Could you check a few things on this model? Use its own coordinates, in mm. Face numbers are marked on the shaded views. Round coordinates to 2 decimals unless told otherwise and drop trailing zeros. Loops run counter-clockwise (first coordinate to the right, second up) from the corner with the lowest first, then second, coordinate; pieces in that order, holes last. Notation, with made-up numbers: (50, 12.25) -> (102, 12.25) arc R19 cw to (102, 40.25) -> close; hole circle Ø4 at (20.25, -36.5). An arc over 180 degrees is marked (long way). One line per item, written item: value.
```python
from build123d import *

# Parameters (mm, degrees)
F0_W     = 67.8
F0_H     = 42
F0_R     = 0.75
F0_W_2   = 2
F0_H_2   = 0.6
F1_DEPTH = 5.3
F2_DEPTH = 1.5
F3_DEPTH = 3.1
F5_DEPTH = 3.3
F7_DEPTH = 1.3
F9_DEPTH = 1.8
F10_SIZE = 0.2


with BuildPart() as f1:
    # F0 (on Top) → F1 (new body)
    with BuildSketch(Plane.XY):
        Rectangle(F0_W, F0_H)
        with Locations((-32.9, -20)):
            Circle(F0_R, mode=Mode.SUBTRACT)
        with Locations((-23.9, -19.7)):
            Rectangle(F0_W_2, F0_H_2, mode=Mode.SUBTRACT)
        with Locations((23.9, -19.7)):
            Rectangle(F0_W_2, F0_H_2, mode=Mode.SUBTRACT)
        with Locations((32.9, -20)):
            Circle(F0_R, mode=Mode.SUBTRACT)
        with Locations((-32.9, 20)):
            Circle(F0_R, mode=Mode.SUBTRACT)
        with Locations((32.9, 20)):
            Circle(F0_R, mode=Mode.SUBTRACT)
        with Locations((32.9, 20)):
            Circle(F0_R)
        with Locations((32.9, -20)):
            Circle(F0_R)
        with Locations((-32.9, 20)):
            Circle(F0_R)
        with Locations((-32.9, -20)):
            Circle(F0_R)
        with Locations((-23.9, -19.7)):
            Rectangle(F0_W_2, F0_H_2)
        with Locations((23.9, -19.7)):
            Rectangle(F0_W_2, F0_H_2)
    extrude(amount=F1_DEPTH)

    # F0 (on Top) → F2 (join)
    with BuildSketch(Plane.XY):
        with Locations((-32.9, -20)):
            Circle(F0_R)
        with Locations((32.9, -20)):
            Circle(F0_R)
        with Locations((32.9, 20)):
            Circle(F0_R)
        with Locations((-32.9, 20)):
            Circle(F0_R)
    extrude(amount=-F2_DEPTH)

    # F0 (on Top) → F3 (join)
    with BuildSketch(Plane.XY):
        with Locations((-23.9, -19.7)):
            Rectangle(F0_W_2, F0_H_2)
        with Locations((23.9, -19.7)):
            Rectangle(F0_W_2, F0_H_2)
    extrude(amount=-F3_DEPTH)

    # F4 (on face) → F5 (cut)
    with BuildSketch(Plane.XY.offset(5.3)):
        Polygon((33, 17), (33, 20), (29.9, 20), (29.9, 21), (-29.9, 21), (-29.9, 20), (-33, 20), (-33, 17), (-33.9, 17), (-33.9, -17), (-33, -17), (-33, -20), (-29.9, -20), (-29.9, -21), (29.9, -21), (29.9, -20), (33, -20), (33, -17), (33.9, -17), (33.9, 17), align=None)
    extrude(amount=-F5_DEPTH, mode=Mode.SUBTRACT)

    # F6 (on face) → F7 (join)
    with BuildSketch(Plane.XY.offset(2)):
        Polygon((33, 17), (33, 20), (29.9, 20), (-29.9, 20), (-33, 20), (-33, 17), (-33, -17), (-33, -20), (-29.9, -20), (29.9, -20), (33, -20), (33, -17), align=None)
    extrude(amount=F7_DEPTH)

    # F8 (on face) → F9 (join)
    with BuildSketch(Plane.XY.offset(3.3)):
        Polygon((-29.9, 20), (-33, 20), (-33, 17), (-33, -13), (33, -13), (33, 17), (33, 20), (29.9, 20), align=None)
    extrude(amount=F9_DEPTH)

    # F10
    f10_edges = [f1.edges().sort_by_distance(p)[0] for p in [
        (-33.65, -20, -1.5),
        (-23.9, -20, -3.1),
        (-22.9, -19.7, -3.1),
        (-23.9, -19.4, -3.1),
        (-24.9, -19.7, -3.1),
        (23.9, -19.4, -3.1),
        (22.9, -19.7, -3.1),
        (23.9, -20, -3.1),
        (24.9, -19.7, -3.1),
        (32.15, -20, -1.5),
        (32.15, 20, -1.5),
        (-33.65, 20, -1.5),
    ]]
    chamfer(f10_edges, length=F10_SIZE)


solid = f1.part
```
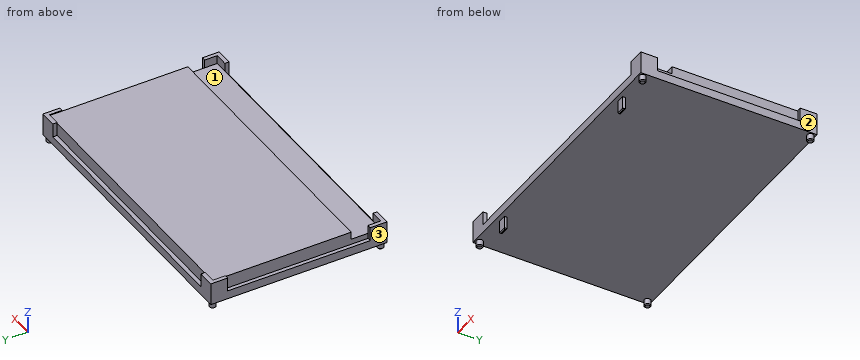
(1) For pin 1 Ø2 at (x, y) = (2, 2.5) entering from +Z; pin 2 Ø12.5 at (x, y) = (-3, -1) entering from -Z; pin 3 Ø0.7 at (y, z) = (-19.5, -1.5) entering from -X, each with a flat end and sliding along its axis, tell me the tip position at first contact or that it passes through.
Results below:
pin 1: stops at z = 5.1
pin 2: stops at z = 0
pin 3: stops at x = -33.62
(2) We'd pull the mould along X, two halves only. Please class the marked faces 1, 2 and 3: +X half, -X half, draft (parallel to the pull), parting line (faces both ways), or undercut.
Results below:
face 1: undercut
face 2: +X half
face 3: -X half
(3) Please list where these lines run through material, in increasing order: L1, parallel to X at y = -19, z = 3.75; L2, parallel to Z at x = 30, y = -12.5; L3, parallel to Y at x = 19.5, z = 5.
Results below:
L1: x = -33.9 to -33, 33 to 33.9
L2: z = 0 to 5.1
L3: y = -13 to 20
(4) Imagine slicing it at A-A on y = -2. Write out the boundary of the cut face in (x, z).
Results below:
outline: (-33.9, 0) -> (33.9, 0) -> (33.9, 2) -> (33, 2) -> (33, 5.1) -> (-33, 5.1) -> (-33, 2) -> (-33.9, 2) -> close
(5) Imagine slicing it at B-B on x = 0. Write out the boundary of the cut face in (y, z).
Results below:
outline: (-21, 0) -> (21, 0) -> (21, 2) -> (20, 2) -> (20, 5.1) -> (-13, 5.1) -> (-13, 3.3) -> (-20, 3.3) -> (-20, 2) -> (-21, 2) -> close
